Could you check a few things on this model? Use its own coordinates, in mm. A direction names the side the tool comes from. Give positions to 0.01 mm unless a question says otherwise; leave off trailing zeros. Loops run counter-clockwise (first coordinate to the right, second up) from the corner with the lowest first, then second, coordinate; pieces in that order, holes last. Notation, with made-up numbers: (52.25, -27.5) - (79.25, -27.5) arc R30 ccw to (79.25, 3.5) - close; hole circle Ø4 at (84, 48.25). An arc over 180 degrees is marked (long way). One line per item, written item: value. Start each with the question number.
Q1. I want a section at C-C (y = 5.5). Please give me the cut outline in (x, z).
Q2. If we mould it in two halves opening along X, with no side actions, what happens to faces 4 (the face through (-1.26, 6.59, 10.01)), 5 (the face through (2, 14, 0)), 6 (the face through (13.887, 12.493, 10.648)), 7 (the face through (-1.5, 7.1, -0.07))? For each: released by +X, released by -X, zero draft, split by the parting line, or undercut.
Q3. If I drill on line 1 (Z direction, x = 0, y = 9.5); line 2 (Z direction, x = 7, y = 11.25); line 3 (X direction, y = 2.5, z = -5.5), over which ranges is the centre line in solid material (lowest first)? Write a range as from..to.
Q4. I want a section at A-A (z = 0). Count the separate pieces of the cut face and the enclosed holes in it, then the cut area to 3 significant figures.
Q5. I'm going to push flat-ended pins straight in: P1, Ø1.5, axis at x = -12, y = 7, coming from the +Z side; P2, Ø6, axis at y = 6.5, z = -10, coming from the -X side (3 decimals); P3, Ø1, axis at x = 9.5, y = 3.5, coming from the +Z side. Where does each tip first touch, or does it pass through?
Q6. For faces 1 (the face through (13.887, 0.493, 10.648)), 2 (the face through (-13.48, 6.59, -0.05)), 3 (the face through (-0.867, 13.493, -3.905)), which set-ups out of +Z, -Z, +X, -X, +Y, -Y let a thin tool reach every point of the face, with its end or its side?
Q7. I want a section at B-B (x = 0). Please give me the cut outline in (y, z).
Autodesk Inventor part; units mm, degrees
ref_plane "Plano de trabajo1" through (0, 1, 0) normal (0, 1, 0) x (-1, 0, 0)
ref_plane "YZ Plane" through (0, 0, 0) normal (1, 0, 0) x (0, 1, 0)
ref_plane "XY Plane" through (0, 0, 0) normal (0, 0, 1) x (1, 0, 0)
sketch "Boceto1" plane through (0, 0, 0) normal (0, 1, 0) x (-1, 0, 0)
  circle A0 centre (0, 0) radius 17.5
  dimension "d0" = 35
extrude "Extrusión1" add sketch "Boceto1" along normal blind 13
sketch "Boceto2" plane through (0, 13, 0) normal (0, 1, 0) x (1, 0, 0)
  circle A0 centre (0, 0) radius 17.5
  circle A1 centre (0, 0) radius 4
  circle A2 centre (0, 10) radius 5
  circle A3 centre (-9.5106, 3.0902) radius 5
  circle A4 centre (-5.8779, -8.0902) radius 5
  circle A5 centre (5.8779, -8.0902) radius 5
  circle A6 centre (9.5106, 3.0902) radius 5
  circle A7 centre (0, 0) radius 17.5
  dimension "d3" = 8
  dimension "d4" = 10
  dimension "d5" = 10
  dimension "d8" = 360
extrude "Extrusión2" add sketch "Boceto2" along normal blind 1 contours A1
extrude "Extrusión3" cut sketch "Boceto2" against normal blind 15 contours A2 | A3 | A4 | A5 | A6
sketch "Boceto3" plane through (0, 14, 0) normal (0, 1, 0) x (1, 0, 0)
  circle A0 centre (0, 0) radius 1.5
  dimension "d14" = 3
extrude "Extrusión4" cut sketch "Boceto3" against normal blind 15
ref_plane "Plano de trabajo1" through (0, 1, 0) normal (0, 1, 0) x (-1, 0, 0)
sketch "Boceto4" plane through (0, 1, 0) normal (0, 1, 0) x (-1, 0, 0)
  circle A0 centre (5.8779, 8.0902) radius 5
  circle A1 centre (-9.5106, -3.0902) radius 5
  circle A2 centre (9.5106, -3.0902) radius 5
  circle A3 centre (0, -10) radius 5
  circle A4 centre (-5.8779, 8.0902) radius 5
  circle A5 centre (0, 0) radius 4
  circle A6 centre (0, 0) radius 17.5
  circle A7 centre (0, 0) radius 20
  dimension "d18" = 40
extrude "Extrusión5" add sketch "Boceto4" along normal blind 11 contours A7
fillet "Empalme1" radius 2 2 edges at (20, 12, 0) (20, 1, 0)
properties part number "Rueda" material "Caucho, butilo(1)"
Worked answers:
1. outline: circle Ø40 at (0, 0); hole circle Ø10 at (-9.51, -3.09); hole circle Ø10 at (-5.88, 8.09); hole circle Ø10 at (0, -10); hole circle Ø3 at (0, 0); hole circle Ø10 at (5.88, 8.09); hole circle Ø10 at (9.51, -3.09)
2. face 4: undercut
2. face 5: zero draft
2. face 6: split by the parting line
2. face 7: undercut
3. line 1: z = -20..-15, -5..-1.5, 1.5..20
3. line 2: z = -18.27..-7.41, 1.23..3.22, 12.96..18.27
3. line 3: x = -19.16..-13.89, -5.13..-2.18, 2.18..5.13, 13.89..19.16
4. separate pieces: 4
4. enclosed holes: 0
4. area: 268 mm²
5. P1: stops at z = 16.54
5. P2: stops at x = -18.735
5. P3: stops at z = 17.86
6. face 1: -Y
6. face 2: +Y, -Y
6. face 3: +Y
7. outline: (0, -17.5) - (1, -17.5) - (1, -18) arc R2 ccw to (3, -20) - (10, -20) arc R2 ccw to (12, -18) - (12, -17.5) - (13, -17.5) - (13, -15) - (0, -15) - close; (0, -5) - (13, -5) - (13, -4) - (14, -4) - (14, -1.5) - (0, -1.5) - close; (0, 1.5) - (14, 1.5) - (14, 4) - (13, 4) - (13, 17.5) - (12, 17.5) - (12, 18) arc R2 ccw to (10, 20) - (3, 20) arc R2 ccw to (1, 18) - (1, 17.5) - (0, 17.5) - close
